Model file for the job. Use its own axes, mm. A direction names the side the tool comes from. Coordinates: 2 decimals unless noted, no trailing zeros. Order: outer loops, then holes, each group sorted by start corner. A loop starts at its lowest first (then second) coordinate and runs counter-clockwise, first axis right, second up. Notation, with made-up numbers: (-10.75, -34.75) -> (26.25, -34.75) arc R17 ccw to (26.25, -10.75) -> close; hole circle Ø5 at (27, 14). An arc over 180 degrees is marked (long way). Return JSON: item names as keys, results as strings. Group by question number.
1) Cut at A-A (y = 14). Write the cut outline in (x, z).
2) Pull direction Y, two halves, no side cores. Call faces 6 (the cylindrical face through (-27.14, 89.1, 0.25)), 7 (the flat face through (-28, 81, 0)), 8 (the flat face through (-17, 44, 17)): +Y half, -Y half, draft (parallel to the pull), parting line (faces both ways), or undercut.
3) Flat gauge pins, fed straight in: pin 1 (3 mm diameter, centred on x = 3.5, z = 8.5, fed in from -Y); pin 2 (3.5 mm diameter, centred on x = -28, z = -9.5, fed in from +Y); pin 3 (2.5 mm diameter, centred on x = 28, z = 0, fed in from +Y); pin 4 (3.5 mm diameter, centred on y = 81, z = 1, fed in from -X). Where does each tip first touch, or does it go through?
4) Probe line 1 (X direction, y = 79.5, z = -14); line 2 (Z direction, x = 2.5, y = 27); line 3 (Z direction, x = 12, y = 72.5). List the from-to ranges inside material, lowest first.
5) Cut at B-B (z = -40.5). Write the cut outline in (x, y).
6) Which spindle directions (+Z, -Z, +X, -X, +Y, -Y) get a long thin tool onto all of the face, cutting with end or side? Do faces 1 (the conical face through (-22.497, 41.709, 22.399)), 2 (the cylindrical face through (27.14, 72.9, -0.25)), 3 (the flat face through (0, 81, -28)), 4 (the cylindrical face through (-11.767, 10.341, -39.86)), 5 (the flat face through (26, 17, 26)). Say none if no direction does.
7) Cut at D-D (y = 58). Write the cut outline in (x, z), and give its area (3 significant figures).
8) Cut at C-C (y = 81). Write the cut outline in (x, z), and give its area (3 significant figures).
from build123d import *

# Parameters (mm, degrees)
BOSS_EXTRUDE1_DEPTH = 38
BOSS_EXTRUDE2_DEPTH = 6
BOSS_EXTRUDE2_TAPER = 45
CUT_EXTRUDE3_START  = -21
CUT_EXTRUDE3_DEPTH  = 78.956123464
CIRPATTERN1_COUNT   = 4
SKETCH5_R           = 3.5
BOSS_EXTRUDE3_DEPTH = 20
BOSS_EXTRUDE4_DEPTH = 18
FILLET1_R           = 3


with BuildPart() as part:
    # Sketch1 → Boss-Extrude1 (new body)
    with BuildSketch(Plane(origin=(0, 0, 0), x_dir=(1, 0, 0), z_dir=(0, 1, 0))):
        with BuildLine():
            Line((-26.5, -30), (26.5, -30))
            ThreePointArc((26.5, -30), (28.974873734, -28.974873734), (30, -26.5))
            Line((30, -26.5), (30, 26.5))
            ThreePointArc((30, 26.5), (28.974873734, 28.974873734), (26.5, 30))
            Line((26.5, 30), (-26.5, 30))
            ThreePointArc((-26.5, 30), (-28.974873734, 28.974873734), (-30, 26.5))
            Line((-30, 26.5), (-30, -26.5))
            ThreePointArc((-30, -26.5), (-28.974873734, -28.974873734), (-26.5, -30))
        make_face()
    extrude(amount=BOSS_EXTRUDE1_DEPTH)

    # Sketch2 → Boss-Extrude2 (add)
    with BuildSketch(Plane(origin=(0, 38, 0), x_dir=(1, 0, 0), z_dir=(0, 1, 0))):
        with BuildLine():
            Line((-18, -28), (18, -28))
            ThreePointArc((18, -28), (25.071067812, -25.071067812), (28, -18))
            Line((28, -18), (28, 18))
            ThreePointArc((28, 18), (25.071067812, 25.071067812), (18, 28))
            Line((18, 28), (-18, 28))
            ThreePointArc((-18, 28), (-25.071067812, 25.071067812), (-28, 18))
            Line((-28, 18), (-28, -18))
            ThreePointArc((-28, -18), (-25.071067812, -25.071067812), (-18, -28))
        make_face()
    extrude(amount=BOSS_EXTRUDE2_DEPTH, taper=BOSS_EXTRUDE2_TAPER)

    # Sketch3 → Cut-Extrude3 (cut)
    with BuildSketch(Plane(origin=(0, 38, 0), x_dir=(1, 0, 0), z_dir=(0, 1, 0)).offset(CUT_EXTRUDE3_START)):
        with BuildLine():
            ThreePointArc((26.660254038, -23), (25.071067812, -25.071067812), (23, -26.660254038))
            Line((23, -26.660254038), (23, -30))
            Line((23, -30), (26.5, -30))
            ThreePointArc((26.5, -30), (28.974873734, -28.974873734), (30, -26.5))
            Line((30, -26.5), (30, -23))
            Line((30, -23), (26.660254038, -23))
        make_face()
        with BuildLine():
            ThreePointArc((26.5, -23), (24.025126266, -24.025126266), (23, -26.5))
            Line((23, -26.5), (23, -26.660254038))
            ThreePointArc((23, -26.660254038), (25.071067812, -25.071067812), (26.660254038, -23))
            Line((26.660254038, -23), (26.5, -23))
        make_face()
    cut_extrude3 = extrude(amount=CUT_EXTRUDE3_DEPTH, mode=Mode.SUBTRACT)

    # CirPattern1: Cut-Extrude3 ×4 about axis
    cirpattern1_axis = Axis((0, 0, 0), (0, 1, 0))
    for i in range(1, CIRPATTERN1_COUNT):
        add(cut_extrude3.rotate(cirpattern1_axis, i * 360 / CIRPATTERN1_COUNT), mode=Mode.SUBTRACT)

    # Sketch4 → Revolve1 (revolve)
    with BuildSketch(Plane.XY, mode=Mode.PRIVATE) as revolve1_sk:
        Polygon((0, 44), (0, 72), (19.550317421, 72), (22, 44), align=None)
    revolve(revolve1_sk.sketch.rotate(Axis((0, -2.2, 0), (0, 1, 0)), 90), axis=Axis((0, -2.2, 0), (0, 1, 0)))

    # Sketch5 → Boss-Extrude3 (add)
    with BuildSketch(Plane(origin=(0, 0, -30), x_dir=(-1, 0, 0), z_dir=(0, 0, -1))):
        with Locations(Location((-15, 9, 0), (0, 0, 180))):
            Circle(SKETCH5_R)
        with Locations(Location((15, 9, 0), (0, 0, 180))):
            Circle(SKETCH5_R)
    extrude(amount=BOSS_EXTRUDE3_DEPTH)

    # Sketch6 → Boss-Extrude4 (add)
    with BuildSketch(Plane(origin=(0, 72, 0), x_dir=(1, 0, 0), z_dir=(0, 1, 0))):
        with BuildLine():
            Line((-18, -28), (18, -28))
            ThreePointArc((18, -28), (25.071067812, -25.071067812), (28, -18))
            Line((28, -18), (28, 18))
            ThreePointArc((28, 18), (25.071067812, 25.071067812), (18, 28))
            Line((18, 28), (-18, 28))
            ThreePointArc((-18, 28), (-25.071067812, 25.071067812), (-28, 18))
            Line((-28, 18), (-28, -18))
            ThreePointArc((-28, -18), (-25.071067812, -25.071067812), (-18, -28))
        make_face()
    extrude(amount=BOSS_EXTRUDE4_DEPTH)

    # Fillet1
    fillet1_edges = [part.edges().sort_by_distance(p)[0] for p in [
        (25.071067812, 72, 25.071067812),
        (28, 72, 0),
        (25.071067812, 72, -25.071067812),
        (0, 72, -28),
        (-25.071067812, 72, -25.071067812),
        (-28, 72, 0),
        (-25.071067812, 72, 25.071067812),
        (0, 72, 28),
        (25.071067812, 90, 25.071067812),
        (28, 90, 0),
        (25.071067812, 90, -25.071067812),
        (0, 90, -28),
        (-25.071067812, 90, -25.071067812),
        (-28, 90, 0),
        (-25.071067812, 90, 25.071067812),
        (0, 90, 28),
    ]]
    fillet(fillet1_edges, radius=FILLET1_R)


solid = part.part
Answers below:
{
 "1": {"outline": "(-30, -26.5) arc R3.5 ccw to (-26.5, -30) -> (26.5, -30) arc R3.5 ccw to (30, -26.5) -> (30, 26.5) arc R3.5 ccw to (26.5, 30) -> (-26.5, 30) arc R3.5 ccw to (-30, 26.5) -> close"},
 "2": {"face 6": "+Y half", "face 7": "draft", "face 8": "undercut"},
 "3": {"pin 1": "stops at y = 0", "pin 2": "stops at y = 89.73", "pin 3": "stops at y = 89.44", "pin 4": "stops at x = -28"},
 "4": {"line 1": "x = -28 to 28", "line 2": "z = -30 to 30", "line 3": "z = -26.66 to 26.66"},
 "5": {"outline": "circle Ø7 at (-15, 9); circle Ø7 at (15, 9)"},
 "6": {"face 1": "+Z, -X", "face 2": "+Z, -Z, +X", "face 3": "-Z, +X, -X, +Y", "face 4": "-Z", "face 5": "+Z, +X"},
 "7": {"outline": "circle Ø41.55 at (0, 0)", "area": "1,360 mm^2"},
 "8": {"outline": "(-28, -18) arc R10 ccw to (-18, -28) -> (18, -28) arc R10 ccw to (28, -18) -> (28, 18) arc R10 ccw to (18, 28) -> (-18, 28) arc R10 ccw to (-28, 18) -> close", "area": "3,050 mm^2"}
}
